The listing builds one solid part. Answer for the finished solid, in the listing's coordinates (mm). Face numbers are marked on the shaded views. Give positions to 0.01 mm unless a question says otherwise; leave off trailing zeros. Loops run counter-clockwise (first coordinate to the right, second up) from the corner with the lowest first, then second, coordinate; pieces in that order, holes last. Notation, with made-up numbers: M -23,-27 L 33,-27 A25 ccw 33,6 Z; hole C 58.25,59 d11. An arc over 180 degrees is marked long. One line per item, written item: value. Start each with the question number.
Q1. Consider L1, parallel to Z at x = 2, y = 5; L2, parallel to Z at x = 1.75, y = 6.5; L3, parallel to Z at x = -4, y = 1.25. Determine where each line is inside the solid, lowest interval first.
Q2. A cutting plane is placed at D-D, the plane z = 0. Determine the outline of the cut face in (x, y) (3 decimals), and give its area (3 significant figures).
Q3. A cutting plane is placed at C-C, the plane y = 5.75. Determine the outline of the cut face in (x, z) (3 decimals), and give its area (3 significant figures).
Q4. The mould has two halves that part along Z. Classify the marked faces 1, 2 and 3: +Z half, -Z half, draft (parallel to the pull), parting line (faces both ways), or undercut.
Q5. A cutting plane is placed at B-B, the plane y = 4.11. Determine the outline of the cut face in (x, z) (3 decimals).
Q6. A flat-ended cylindrical pin translates along its axis: pin 1 (2.5 mm diameter, centred on y = 4.11, z = 7.36, fed in from -X) (3 decimals). Find the tip coordinate at first contact, or state that the pin passes through.
Q7. A cutting plane is placed at A-A, the plane x = 0. State how many separate pieces and enclosed holes the cut face has, and give its area (3 significant figures).
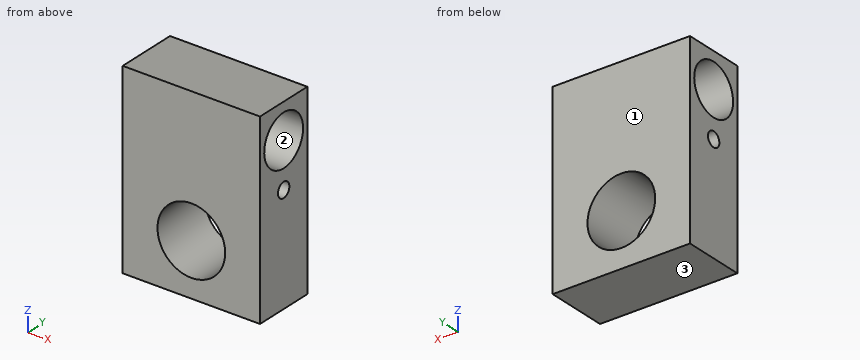
from build123d import *

# Parameters (mm, degrees)
SKETCH1_W              = 18.25
SKETCH1_H              = 25
BOSS_EXTRUDE1_DEPTH    = 8.22
M10X1_0_TAPPED_HOLE1_D = 9
SKETCH7_R              = 3.375
SKETCH7_R_2            = 0.9906
CUT_EXTRUDE2_DEPTH     = 19.25


with BuildPart() as part:
    # Sketch1 → Boss-Extrude1 (new body)
    with BuildSketch(Plane(origin=(0, 0, 0), x_dir=(1, 0, 0), z_dir=(0, 1, 0))):
        with Locations((0, -5.5)):
            Rectangle(SKETCH1_W, SKETCH1_H)
    extrude(amount=BOSS_EXTRUDE1_DEPTH)

    # M10x1.0 Tapped Hole1 (through all)
    with Locations(Plane(origin=(0, 8.22, 0), x_dir=(-1, 0, 0), z_dir=(0, 1, 0))):
        with Locations((0, 0)):
            Hole(M10X1_0_TAPPED_HOLE1_D / 2)

    # Sketch7 → Cut-Extrude2 (cut, through all)
    with BuildSketch(Plane(origin=(9.125, 0, 0), x_dir=(0, 0, -1), z_dir=(1, 0, 0))):
        with Locations((-13.336186812, 4.11)):
            Circle(SKETCH7_R)
        with Locations((-7.3575, 4.11)):
            Circle(SKETCH7_R_2)
    extrude(amount=-CUT_EXTRUDE2_DEPTH, mode=Mode.SUBTRACT)


solid = part.part
Answer block:
1. L1: -7 to -4.03, 4.03 to 6.92, 7.79 to 10.08, 16.59 to 18
1. L2: -7 to -4.15, 4.15 to 10.95, 15.72 to 18
1. L3: -7 to -2.06, 2.06 to 11.54, 15.13 to 18
2. outline: M -9.125,0 L -4.5,0 L -4.5,8.22 L -9.125,8.22 Z; M 4.5,0 L 9.125,0 L 9.125,8.22 L 4.5,8.22 Z
2. area: 76.0 mm^2
3. outline: M -9.125,-7 L 9.125,-7 L 9.125,10.386 L -9.125,10.386 Z; M -9.125,16.286 L 9.125,16.286 L 9.125,18 L -9.125,18 Z; hole C 0,0 d9
3. area: 285 mm^2
4. face 1: draft
4. face 2: undercut
4. face 3: -Z half
5. outline: M -9.125,-7 L 9.125,-7 L 9.125,6.367 L -9.125,6.367 Z; M -9.125,8.348 L 9.125,8.348 L 9.125,9.961 L -9.125,9.961 Z; M -9.125,16.711 L 9.125,16.711 L 9.125,18 L -9.125,18 Z; hole C 0,0 d9
6. pin 1: x = -9.125
7. separate pieces: 2
7. enclosed holes: 2
7. area: 92.7 mm^2
